The listing builds one solid part. Answer for the finished solid, in the listing's coordinates (mm). Face numbers are marked on the shaded views. A direction names the side the tool comes from. Give positions to 0.01 mm unless a question says otherwise; leave off trailing zeros. Loops run counter-clockwise (first coordinate to the right, second up) from the corner with the lowest first, then second, coordinate; pieces in that order, holes last. Notation, with made-up numbers: M -38.75,62 L -12.75,62 A24 ccw -12.75,72 Z; hole C 31,41 d8. An arc over 180 degrees is marked long. One line per item, written item: value. Start each with the question number.
Q1. A cutting plane is placed at B-B, the plane y = -18.5. Determine the outline of the cut face in (x, z), and give its area (3 significant figures).
Q2. Consider L1, parallel to Y at x = 0, z = 4; L2, parallel to Z at x = 20, y = 7.5; L3, parallel to Z at x = 2.5, y = -13. Determine where each line is inside the solid, lowest interval first.
Q3. A cutting plane is placed at A-A, the plane y = -9.5. Determine the outline of the cut face in (x, z), and give its area (3 significant figures).
Q4. The mould has two halves that part along X. Classify the marked faces 3, 4 and 5: +X half, -X half, draft (parallel to the pull), parting line (faces both ways), or undercut.
Q5. Flat-ended cylindrical pins translate along their axes: pin 1 (7.5 mm diameter, centred on x = 6.5, z = 13.5, fed in from -Y); pin 2 (3 mm diameter, centred on x = 7.5, z = 11, fed in from +Y); pin 3 (1.5 mm diameter, centred on x = 3.5, y = -10, fed in from +Z). Find the tip coordinate at first contact, or state that the pin passes through.
Q6. For the marked faces 1 and 2, determine the directions among +Z, -Z, +X, -X, +Y, -Y from which every point of the face is accessible in a straight line to the end or side of a thin tool.
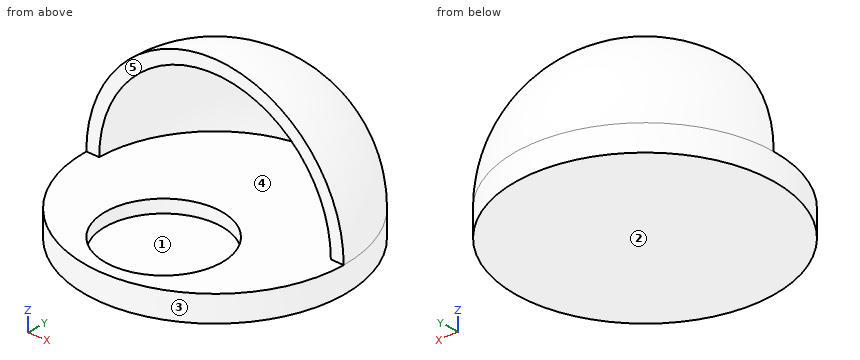
from build123d import *

# Parameters (mm, degrees)
F0_R     = 25.4
F0_R_2   = 11.43
F1_DEPTH = 5.08
F2_DEPTH = 2.54
F4_ANGLE = 180


with BuildPart() as f1:
    # F0 (on Top) → F1 (new body)
    with BuildSketch(Plane.XY):
        Circle(F0_R)
        with Locations((0, -11.43)):
            Circle(F0_R_2, mode=Mode.SUBTRACT)
    extrude(amount=F1_DEPTH)

    # F0 (on Top) → F2 (join)
    with BuildSketch(Plane.XY):
        with Locations((0, -11.43)):
            Circle(F0_R_2)
    extrude(amount=F2_DEPTH)

    # F3 (on face) → F4 (revolve)
    with BuildSketch(Plane.XY.offset(5.08)):
        with BuildLine():
            Line((22.86, 0), (25.4, 0))
            ThreePointArc((25.4, 0), (17.960512, 17.960512), (0, 25.4))
            Line((0, 25.4), (0, 22.86))
            ThreePointArc((0, 22.86), (16.164461, 16.164461), (22.86, 0))
        make_face()
    revolve(axis=Axis((0, 24.13, 5.08), (0, -1, 0)), revolution_arc=F4_ANGLE)


solid = f1.part
Answer block:
1. outline: M -17.4,0 L 17.4,0 L 17.4,5.08 L 8.98,5.08 L 8.98,2.54 L -8.98,2.54 L -8.98,5.08 L -17.4,5.08 Z
1. area: 131 mm^2
2. L1: -25.4 to -22.86, 0 to 25.4
2. L2: 0 to 5.08, 13.22 to 18.82
2. L3: 0 to 2.54
3. outline: M -23.56,0 L 23.56,0 L 23.56,5.08 L 11.27,5.08 L 11.27,2.54 L -11.27,2.54 L -11.27,5.08 L -23.56,5.08 Z
3. area: 182 mm^2
4. face 3: parting line
4. face 4: undercut
4. face 5: draft
5. pin 1: y = 17.76
5. pin 2: y = 24.09
5. pin 3: z = 2.54
6. face 1: +Z
6. face 2: -Z, +X, -X, +Y, -Y
